```python
from build123d import *

# Parameters (mm, degrees)
F0_R     = 4.9022
F1_DEPTH = 3.175


with BuildPart() as f1:
    # F0 (on Top) → F1 (new body)
    with BuildSketch(Plane.XY):
        with BuildLine():
            Line((43.214022, 26.049825), (0.008622, -48.784123))
            Line((0.008622, -48.784123), (0.005029, -56.721344))
            ThreePointArc((0.005029, -56.721344), (1.127097, -57.186566), (1.591811, -58.308844))
            ThreePointArc((1.591811, -58.308844), (1.126589, -59.43163), (0.003592, -59.896344))
            Line((0.003592, -59.896344), (0, -67.833564))
            Line((0, -67.833564), (119.414022, -67.833564))
            Line((119.414022, -67.833564), (59.711322, 35.574545))
            Line((59.711322, 35.574545), (52.837487, 31.605935))
            ThreePointArc((52.837487, 31.605935), (52.996079, 31.22306), (53.050172, 30.812185))
            ThreePointArc((53.050172, 30.812185), (51.873547, 29.278778), (50.087856, 30.018435))
            Line((50.087856, 30.018435), (43.214022, 26.049825))
        make_face()
        with BuildLine():
            Line((-50.070613, 30.018435), (-43.196778, 26.049825))
            Line((-43.196778, 26.049825), (43.214022, 26.049825))
            Line((43.214022, 26.049825), (50.087856, 30.018435))
            ThreePointArc((50.087856, 30.018435), (50.668922, 32.187), (52.837487, 31.605935))
            Line((52.837487, 31.605935), (59.711322, 35.574545))
            Line((59.711322, 35.574545), (0.008622, 138.982655))
            Line((0.008622, 138.982655), (-59.694078, 35.574545))
            Line((-59.694078, 35.574545), (-52.820244, 31.605935))
            ThreePointArc((-52.820244, 31.605935), (-51.034553, 32.345592), (-49.857928, 30.812185))
            ThreePointArc((-49.857928, 30.812185), (-49.912021, 30.40131), (-50.070613, 30.018435))
        make_face()
        with BuildLine():
            Line((0.008622, -48.784123), (-43.196778, 26.049825))
            Line((-43.196778, 26.049825), (-50.070613, 30.018435))
            ThreePointArc((-50.070613, 30.018435), (-52.239178, 29.43737), (-52.820244, 31.605935))
            Line((-52.820244, 31.605935), (-59.694078, 35.574545))
            Line((-59.694078, 35.574545), (-119.396778, -67.833564))
            Line((-119.396778, -67.833564), (0, -67.833564))
            Line((0, -67.833564), (0.003592, -59.896344))
            ThreePointArc((0.003592, -59.896344), (-1.583189, -58.308125), (0.005029, -56.721344))
            Line((0.005029, -56.721344), (0.008622, -48.784123))
        make_face()
        Polygon((-63.696348, -65.656609), (-63.696348, -63.431569), (-63.696348, -61.206529), (-55.700428, -61.206529), (-55.700428, -63.431569), (-55.700428, -65.656609), align=None, mode=Mode.SUBTRACT)
        Polygon((-61.476388, -56.827569), (-61.476388, -52.255569), (-61.476388, -47.683569), (-57.920388, -47.683569), (-57.920388, -52.255569), (-57.920388, -56.827569), align=None, mode=Mode.SUBTRACT)
        with Locations((-59.698388, -40.190569)):
            Circle(F0_R, mode=Mode.SUBTRACT)
    extrude(amount=F1_DEPTH)


solid = f1.part
```
Input: part model. Units: mm. Frame: model coordinates. A direction names the side the tool comes from. Round coordinates to 2 decimals unless told otherwise and drop trailing zeros. Loops run counter-clockwise (first coordinate to the right, second up) from the corner with the lowest first, then second, coordinate; pieces in that order, holes last. Notation, with made-up numbers: (58.5, 16) - (73.5, 16) arc R14 cw to (73.5, 28) - close; hole circle Ø1 at (7.25, 42.5). An arc over 180 degrees is marked (long way). One line per item, written item: value. Start each with the question number.
(1) Access query for faces 1 (the flat face through (-28, -9, 0)), 2 (the flat face through (21.914, -10.843, 1.565)). Directions: +Z, -Z, +X, -X, +Y, -Y. A direction counts if a zero-diameter tool reaches every point of the face in a straight line with its end or side. Return the directions, or none.
(2) Section A-A, the plane x = -24. Return loops of the section in (y, z) (1 decimal), plus the area to 3 significant figures.
(3) Section C-C, the plane y = -14.5. Return loops of the section in (x, z) (3 decimals), plus the area to 3 significant figures.
(4) Contact query for flat-ended pins moving along their axis: P1, Ø1, axis at y = -44.5, z = 2.5, coming from the -X side; P2, Ø1.6, axis at y = -50, z = 1, coming from the -X side; P3, Ø1.6, axis at x = -59, z = 1, coming from the +Y side; P4, Ø5, axis at x = 36.5, y = 7, coming from the -Z side. Output: stop coordinate, or through.
(5) Draft query along X for faces 3 (the flat face through (-28, -9, 3.175)), 4 (the flat face through (-21.29, -11.89, 1.57)). Return one class per face: +X half, -X half, draft (parallel to the pull), parting line (faces both ways), or undercut.
(6) Section B-B, the plane z = 1.95. Return loops of the section in (x, y) (1 decimal), plus the area to 3 significant figures.
(7) Ray query, line 1 (Y direction, x = 40.5, z = 0.25); line 2 (X direction, y = 32, z = 0.95); line 3 (Y direction, x = -42, z = 2.85). Return the intervals inside material, ascending. Write a range as [from, to].
(8) Section D-D, the plane y = 40. Return loops of the section in (x, z) (3 decimals), plus the area to 3 significant figures.
Results below:
1. face 1: -Z, +X, -X, +Y, -Y
1. face 2: +Z, -Z
2. outline: (-67.8, 0) - (-7.2, 0) - (-7.2, 3.2) - (-67.8, 3.2) - close; (26, 0) - (97.4, 0) - (97.4, 3.2) - (26, 3.2) - close
2. area: 419 mm^2
3. outline: (-88.605, 0) - (-19.785, 0) - (-19.785, 3.175) - (-88.605, 3.175) - close; (19.803, 0) - (88.622, 0) - (88.622, 3.175) - (19.803, 3.175) - close
3. area: 437 mm^2
4. P1: x = -106.21
4. P2: x = -109.56
4. P3: y = 38.16
4. P4: z = 0
5. face 3: draft
5. face 4: undercut
6. outline: (-119.4, -67.8) - (119.4, -67.8) - (0, 139) - close; hole circle Ø9.8 at (-59.7, -40.2); hole (-63.7, -65.7) - (-55.7, -65.7) - (-55.7, -61.2) - (-63.7, -61.2) - close; hole (-61.5, -56.8) - (-57.9, -56.8) - (-57.9, -47.7) - (-61.5, -47.7) - close; hole (-52.8, 31.6) arc R1.6 ccw to (-50.1, 30) arc R1.6 ccw to (-49.9, 30.8) arc R1.6 ccw to start; hole (-43.2, 26) - (0, -48.8) - (43.2, 26) - close; hole circle Ø3.2 at (0, -58.3); hole (50.1, 30) arc R1.6 ccw to (53.1, 30.8) arc R1.6 ccw to (52.8, 31.6) arc R1.6 ccw to start
6. area: 21,300 mm^2
7. line 1: [-67.83, 21.35], [26.05, 68.85]
7. line 2: [-61.76, -52.5], [-50.39, 50.41], [52.52, 61.78]
7. line 3: [-67.83, 23.98], [26.05, 66.22]
8. outline: (-57.139, 0) - (57.156, 0) - (57.156, 3.175) - (-57.139, 3.175) - close
8. area: 363 mm^2
